from build123d import *

# Parameters (mm, degrees)
REVOLUTION003_ANGLE = 180
PAD021_DEPTH        = 5.25
FILLET004_R         = 0.49
PAD022_DEPTH        = 0.2


with BuildPart() as part:
    # Sketch038 → Revolution003 (revolve)
    with BuildSketch(Plane.XZ):
        with BuildLine():
            Line((5.25, 2.7), (5.25, 2.2))
            Line((5.25, 2.2), (5.95, 2.2))
            Line((5.95, 2.2), (5.95, 0.45))
            ThreePointArc((5.95, 0.45), (6.2, 0.2), (6.45, 0.45))
            Line((6.45, 0.45), (6.45, 2.2))
            ThreePointArc((6.45, 2.2), (6.3035533906, 2.5535533906), (5.95, 2.7))
            Line((5.25, 2.7), (5.95, 2.7))
        make_face()
    revolve(axis=Axis((0, 0, 0), (0, 0, 1)), revolution_arc=REVOLUTION003_ANGLE)

    # Sketch038 → Pad021 (new body)
    with BuildSketch(Plane.XZ):
        with BuildLine():
            Line((5.25, 2.7), (5.25, 2.2))
            Line((5.25, 2.2), (5.95, 2.2))
            Line((5.95, 2.2), (5.95, 0.45))
            ThreePointArc((5.95, 0.45), (6.2, 0.2), (6.45, 0.45))
            Line((6.45, 0.45), (6.45, 2.2))
            ThreePointArc((6.45, 2.2), (6.3035533906, 2.5535533906), (5.95, 2.7))
            Line((5.25, 2.7), (5.95, 2.7))
        make_face()
    pad021 = extrude(amount=PAD021_DEPTH)

    # Mirrored: Pad021 across Sketch038 V_Axis
    add(pad021.mirror(Plane(origin=(0, 0, 0), x_dir=(0, -1, 0), z_dir=(1, 0, 0))))

    # Fillet004
    fillet004_edges = [part.edges().sort_by_distance(p)[0] for p in [
        (-5.25, -5.25, 2.45),
        (5.25, -5.25, 2.45),
    ]]
    fillet(fillet004_edges, radius=FILLET004_R)

    # Sketch045 → Pad022 (join)
    with BuildSketch(Plane.XY.offset(2.7)):
        with BuildLine():
            ThreePointArc((-1.9419855366, 8.5580144634), (0, 7.0362321709), (1.9419855366, 8.5580144634))
            ThreePointArc((5.25, 5.25), (4.2811049959, 7.5891194594), (1.9419855366, 8.5580144634))
            Line((5.25, 5.25), (5.25, 2.8))
            ThreePointArc((5.95, 0), (5.7723478759, 1.443086969), (5.25, 2.8))
            Line((5.95, 0), (5.95, 5.25))
            ThreePointArc((5.95, 5.25), (4.7921943754, 8.0678874204), (1.9876941818, 9.2577538171))
            ThreePointArc((1.9876941818, 9.2577538172), (0, 11.0362321709), (-1.9876941818, 9.2577538172))
            ThreePointArc((-1.9876941818, 9.2577538171), (-4.7921943754, 8.0678874204), (-5.95, 5.25))
            Line((-5.95, 0), (-5.95, 5.25))
            ThreePointArc((-5.25, 2.8), (-5.7723478759, 1.443086969), (-5.95, 0))
            Line((-5.25, 5.25), (-5.25, 2.8))
            ThreePointArc((-1.9419855366, 8.5580144634), (-4.2811049959, 7.5891194594), (-5.25, 5.25))
        make_face()
    extrude(amount=-PAD022_DEPTH)


solid = part.part
Verification items for the finished model (mm, model axes). A direction names the side the tool comes from. Give positions to 0.01 mm unless a question says otherwise; leave off trailing zeros. Write each loop counter-clockwise with the first axis right and the second up, starting at its lowest first coordinate (ties: lowest second). Pieces come first, ordered by that corner, then holes.
(1) Cross-section at B-B (x = 0). Enter the section's corners in (y, z), plus the area to 3 significant figures.
(2) Cross-section at A-A (y = -2.25). Enter the section's corners in (x, z), plus the area to 3 significant figures.
(3) Access from +Z, -Z, +X, -X, +Y, -Y to the whole of each face (thin tool, end or side, straight path). Record for faces 1 (the face through (6.45, -3, 1)), 2 (the face through (5.95, -3, 1)).
(4) Cross-section at C-C (y = 5.5). State how many separate pieces and enclosed holes the cut face has, plus the area to 3 significant figures.
(5) Mould release check, pull along X, two halves, no side actions. Record for faces 3 (the face through (0.13, 5.95, 1.31)), 4 (the face through (0.14, 6.45, 1.34)), 5 (the face through (1.3, 5.3, 2.7)): +X half, -X half, draft (parallel to the pull), parting line (faces both ways), or undercut.
(6) Material ranges on line 1 (X direction, y = -2.5, z = 1.55); line 2 (X direction, y = 3.75, z = 1.45); line 3 (Z direction, x = -5.75, y = -4.25), recorded low to high.
(7) Gauge pin test, flat end, axial feed: pin 1 (4.5 mm diameter, centred on x = 1, y = 9, fed in from -Z). Record the tip position at first contact, or that the pin passes through.
Worked out:
1. outline: (5.25, 2.2) - (5.95, 2.2) - (5.95, 0.45) arc R0.25 ccw to (6.45, 0.45) - (6.45, 2.2) arc R0.5 ccw to (5.95, 2.7) - (5.25, 2.7) - close; (7.04, 2.5) - (11.04, 2.5) - (11.04, 2.7) - (7.04, 2.7) - close
1. area: 2.32 mm2
2. outline: (-6.45, 0.45) arc R0.25 ccw to (-5.95, 0.45) - (-5.95, 2.2) - (-5.25, 2.2) - (-5.25, 2.7) - (-5.95, 2.7) arc R0.5 ccw to (-6.45, 2.2) - close; (5.25, 2.2) - (5.95, 2.2) - (5.95, 0.45) arc R0.25 ccw to (6.45, 0.45) - (6.45, 2.2) arc R0.5 ccw to (5.95, 2.7) - (5.25, 2.7) - close
2. area: 3.04 mm2
3. face 1: +Z, -Z, +X, +Y, -Y
3. face 2: -Z, -Y
4. separate pieces: 3
4. enclosed holes: 0
4. area: 7.71 mm2
5. face 3: undercut
5. face 4: parting line
5. face 5: draft
6. line 1: x = -6.45 to -5.95, 5.95 to 6.45
6. line 2: x = -5.25 to -4.62, 4.62 to 5.25
6. line 3: z = 2.2 to 2.7
7. pin 1: stops at z = 2.5
